```python
from build123d import *

# Parameters (mm, degrees)
SKETCH1_R                                     = 10.8
EXTRUDE1_DEPTH                                = 0.75
SKETCH2_R                                     = 10.6
EXTRUDE2_DEPTH                                = 5.5
EXTRUDE3_START                                = 5.5
SKETCH3_R                                     = 10.6
EXTRUDE3_DEPTH                                = 5.5
SKETCH4_W                                     = 16
SKETCH4_H                                     = 9
EXTRUDE4_DEPTH                                = 2
SKETCH5_W                                     = 13.3
SKETCH5_H                                     = 5.75
EXTRUDE5_DEPTH                                = 10.8
EXTRUDE6_DEPTH                                = 10.8
SKETCH7_W                                     = 10.8
SKETCH7_H                                     = 1.3
EXTRUDE7_DEPTH                                = 10.5
CHAMFER1_SIZE                                 = 0.25
SKETCH8_W                                     = 11
SKETCH8_H                                     = 12
EXTRUDE8_DEPTH                                = 13.15
EXTRUDE9_DEPTH                                = 13.15
SKETCH10_W                                    = 5.5
SKETCH10_H                                    = 3
EXTRUDE10_DEPTH                               = 13
CHAMFER2_SIZE                                 = 0.25
EXTRUDE11_DEPTH                               = 30.552834043
SKETCH12_R                                    = 10.15
EXTRUDE12_DEPTH                               = 1.25
EXTRUDE13_DEPTH                               = 13
EXTRUDE13_DEPTH_BACK                          = 5
SKETCH13_R                                    = 11.75
SKETCH13_R_2                                  = 10.15
SKETCH14_W                                    = 26
SKETCH14_H                                    = 31
SKETCH14_R                                    = 11.75
EXTRUDE14_DEPTH                               = 2
CSK_FOR_M3_COUNTERSUNK_FLAT_HEAD1_D           = 3.2
CSK_FOR_M3_COUNTERSUNK_FLAT_HEAD1_CSINK_D     = 6.3
CSK_FOR_M3_COUNTERSUNK_FLAT_HEAD1_CSINK_ANGLE = 90
FILLET1_R                                     = 3


with BuildPart() as part:
    # Sketch1 → Extrude1 (new, symmetric)
    with BuildSketch(Plane.XY):
        Circle(SKETCH1_R)
    extrude(amount=EXTRUDE1_DEPTH, both=True)

    # Sketch2 → Extrude2 (add)
    with BuildSketch(Plane.XY.offset(0.75)):
        Circle(SKETCH2_R)
    extrude(amount=EXTRUDE2_DEPTH)

    # Sketch3 → Extrude3 (add)
    with BuildSketch(Plane(origin=(0, 0, -0.75), x_dir=(-1, 0, 0), z_dir=(0, 0, -1)).offset(EXTRUDE3_START)):
        with Locations(Location((0, 0, 0), (0, 0, 180))):
            Circle(SKETCH3_R)
    extrude(amount=-EXTRUDE3_DEPTH)

    # Sketch4 → Extrude4 (add)
    with BuildSketch(Plane.XY.offset(6.25)):
        Rectangle(SKETCH4_W, SKETCH4_H)
    extrude(amount=EXTRUDE4_DEPTH)

    # Sketch5 → Extrude5 (add)
    with BuildSketch(Plane.XY.offset(8.25)):
        Rectangle(SKETCH5_W, SKETCH5_H)
    extrude(amount=EXTRUDE5_DEPTH)

    # Sketch6 → Extrude6 (cut)
    with BuildSketch(Plane.XY.offset(19.05)):
        Polygon((-5.9, 2.625), (5.9, 2.625), (6.4, 2.125), (6.4, -2.125), (5.9, -2.625), (-5.9, -2.625), (-6.4, -2.125), (-6.4, 2.125), align=None)
    extrude(amount=-EXTRUDE6_DEPTH, mode=Mode.SUBTRACT)

    # Sketch7 → Extrude7 (add)
    with BuildSketch(Plane.XY.offset(8.25)):
        with Locations((0, 0.975)):
            Rectangle(SKETCH7_W, SKETCH7_H)
    extrude(amount=EXTRUDE7_DEPTH)

    # Chamfer1
    chamfer1_edges = [part.edges().sort_by_distance(p)[0] for p in [
        (-5.4, 0.975, 18.75),
        (0, 0.325, 18.75),
        (5.4, 0.975, 18.75),
        (0, 1.625, 18.75),
    ]]
    chamfer(chamfer1_edges, length=CHAMFER1_SIZE)

    # Sketch8 → Extrude8 (add)
    with BuildSketch(Plane(origin=(0, 0, -6.25), x_dir=(-1, 0, 0), z_dir=(0, 0, -1))):
        Rectangle(SKETCH8_W, SKETCH8_H)
    extrude(amount=EXTRUDE8_DEPTH)

    # Sketch9 → Extrude9 (cut)
    with BuildSketch(Plane(origin=(0, 0, -19.4), x_dir=(-1, 0, 0), z_dir=(0, 0, -1))):
        Polygon((-2.85, 4.6), (2.85, 4.6), (3.85, 3.6), (3.85, -4.35), (-3.85, -4.35), (-3.85, 3.6), align=None)
    extrude(amount=-EXTRUDE9_DEPTH, mode=Mode.SUBTRACT)

    # Sketch10 → Extrude10 (add)
    with BuildSketch(Plane(origin=(0, 0, -6.25), x_dir=(-1, 0, 0), z_dir=(0, 0, -1))):
        Rectangle(SKETCH10_W, SKETCH10_H)
    extrude(amount=EXTRUDE10_DEPTH)

    # Chamfer2
    chamfer2_edges = [part.edges().sort_by_distance(p)[0] for p in [
        (2.75, 0, -19.25),
        (0, -1.5, -19.25),
        (-2.75, 0, -19.25),
        (0, 1.5, -19.25),
    ]]
    chamfer(chamfer2_edges, length=CHAMFER2_SIZE)

    # Sketch11 → Extrude11 (cut, through all)
    with BuildSketch(Plane(origin=(0, 0, -6.25), x_dir=(-1, 0, 0), z_dir=(0, 0, -1))):
        with BuildLine():
            Line((-2.75, 10), (-2.75, 10.444017426))
            ThreePointArc((-2.75, 10.444017426), (0, 10.8), (2.75, 10.444017426))
            Line((2.75, 10.444017426), (2.75, 10))
            ThreePointArc((2.75, 10), (0, 7.25), (-2.75, 10))
        make_face()
        with BuildLine():
            Line((-2.75, -10.444017426), (-2.75, -10))
            ThreePointArc((-2.75, -10), (0, -7.25), (2.75, -10))
            Line((2.75, -10), (2.75, -10.444017426))
            ThreePointArc((2.75, -10.444017426), (0, -10.8), (-2.75, -10.444017426))
        make_face()
    extrude(amount=-EXTRUDE11_DEPTH, mode=Mode.SUBTRACT)

    # Sketch12 → Extrude12 (add)
    with BuildSketch(Plane.XY.offset(6.25)):
        with Locations(Location((0, 0, 0), (0, 0, 105.664941507))):
            Circle(SKETCH12_R)
        Polygon((7.3, 4.8), (8.3, 4.8), (8.3, -4.8), (7.3, -4.8), (7.3, -5.25), (-7.3, -5.25), (-7.3, -4.8), (-8.3, -4.8), (-8.3, 4.8), (-7.3, 4.8), (-7.3, 5.25), (7.3, 5.25), align=None, mode=Mode.SUBTRACT)
    extrude(amount=EXTRUDE12_DEPTH)

    # Sketch13 → Extrude13 (add, two sides: drawn at the far end of the back side and taken through both)
    with BuildSketch(Plane.XY.offset(7.5).offset(-EXTRUDE13_DEPTH_BACK)):
        Circle(SKETCH13_R)
        Circle(SKETCH13_R_2, mode=Mode.SUBTRACT)
    extrude(amount=EXTRUDE13_DEPTH + EXTRUDE13_DEPTH_BACK)

    # Sketch14 → Extrude14 (add)
    with BuildSketch(Plane.XY.offset(17.65)):
        Rectangle(SKETCH14_W, SKETCH14_H)
        Circle(SKETCH14_R, mode=Mode.SUBTRACT)
    extrude(amount=-EXTRUDE14_DEPTH)

    # CSK for M3 Countersunk Flat Head1 (through all)
    with Locations(Plane.XY.offset(17.65)):
        with Locations((-9.5, 12), (9.5, -12)):
            CounterSinkHole(CSK_FOR_M3_COUNTERSUNK_FLAT_HEAD1_D / 2, CSK_FOR_M3_COUNTERSUNK_FLAT_HEAD1_CSINK_D / 2, counter_sink_angle=CSK_FOR_M3_COUNTERSUNK_FLAT_HEAD1_CSINK_ANGLE)

    # Fillet1
    fillet1_edges = [part.edges().sort_by_distance(p)[0] for p in [
        (-13, -15.5, 16.65),
        (-13, 15.5, 16.65),
        (13, 15.5, 16.65),
        (13, -15.5, 16.65),
    ]]
    fillet(fillet1_edges, radius=FILLET1_R)


solid = part.part
```
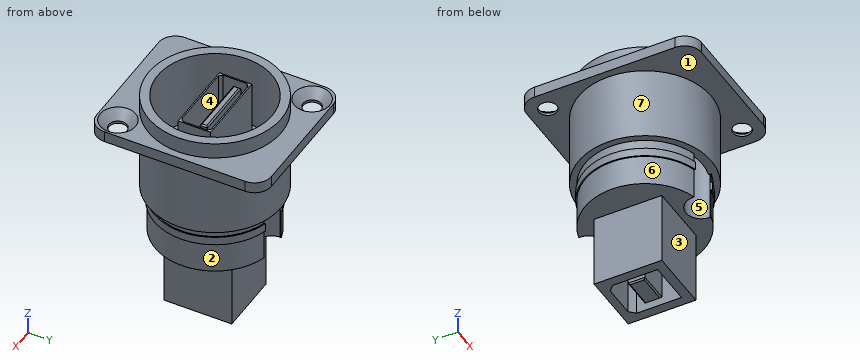
The model under review builds one solid part; all positions refer to its coordinate system, in mm. Face numbers are marked on the shaded views. A direction names the side the tool comes from. Round coordinates to 2 decimals unless told otherwise and drop trailing zeros. Order: outer loops, then holes, each group sorted by start corner. A loop starts at its lowest first (then second) coordinate and runs counter-clockwise, first axis right, second up.
(1) Take a section at A-A, the plane z = 9.5. State the section outline as (x, y) points (3 decimals).
Working result:
outline: circle Ø23.5 at (0, 0); (-6.65, -2.875) - (6.65, -2.875) - (6.65, 2.875) - (-6.65, 2.875) - close; (-5.4, 0.325) - (5.4, 0.325) - (5.4, 1.625) - (-5.4, 1.625) - close; hole circle Ø20.3 at (0, 0); hole (-6.4, -2.125) - (-5.9, -2.625) - (5.9, -2.625) - (6.4, -2.125) - (6.4, 2.125) - (5.9, 2.625) - (-5.9, 2.625) - (-6.4, 2.125) - close
(2) Take a section at B-B, the plane z = -10.5. State the section outline as (x, y) points.
Working result:
outline: (-5.5, -6) - (5.5, -6) - (5.5, 6) - (-5.5, 6) - close; (-2.75, -1.5) - (2.75, -1.5) - (2.75, 1.5) - (-2.75, 1.5) - close; hole (-3.85, -4.35) - (3.85, -4.35) - (3.85, 3.6) - (2.85, 4.6) - (-2.85, 4.6) - (-3.85, 3.6) - close
(3) For P1, Ø1.5, axis at x = 0, z = -12, coming from the -Y side; P2, Ø1.5, axis at x = 3, y = 7, coming from the +Z side; P3, Ø3, axis at x = 0, y = -9, coming from the -Z side, all flat-tipped, find the tip position at first contact; note any pin that passes through.
Working result:
P1: stops at y = -6
P2: stops at z = 7.5
P3: stops at z = 2.5
(4) Take a section at D-D, the plane y = -6.5. State the section outline as (x, z) points.
Working result:
outline: (-13, 15.65) - (-9.79, 15.65) - (-9.79, 2.5) - (-8.37, 2.5) - (-8.37, 0.75) - (-8.62, 0.75) - (-8.62, -0.75) - (-8.37, -0.75) - (-8.37, -6.25) - (8.37, -6.25) - (8.37, -0.75) - (8.62, -0.75) - (8.62, 0.75) - (8.37, 0.75) - (8.37, 2.5) - (9.79, 2.5) - (9.79, 15.65) - (13, 15.65) - (13, 17.65) - (9.79, 17.65) - (9.79, 20.5) - (7.8, 20.5) - (7.8, 7.5) - (-7.8, 7.5) - (-7.8, 20.5) - (-9.79, 20.5) - (-9.79, 17.65) - (-13, 17.65) - close
(5) Tool access review of the marked faces 1, 2, 3 and 4: name each direction out of +Z, -Z, +X, -X, +Y, -Y from which nothing blocks a thin tool from reaching the whole face with its end or side.
Working result:
face 1: -Z
face 2: -Z, +X
face 3: -Z, +X, -X, -Y
face 4: +Z
(6) Wall thickness on L1, parallel to Y at x = -0.5, z = 6.5; L2, parallel to Y at x = 1.75, z = 17.5 (3 decimals); L3, parallel to Y at x = 5, z = 7: over which ranges is each line inside the solid? List them lowest first.
Working result:
L1: y = -11.74 to -5.25, -4.5 to 4.5, 5.25 to 11.74
L2: y = -15.5 to -9.998, -2.875 to -2.625, 0.325 to 1.625, 2.625 to 2.875, 9.998 to 15.5
L3: y = -10.63 to -5.25, -4.5 to 4.5, 5.25 to 10.63
(7) Mouldability with a two-part tool opening along X and no side actions: class the marked faces 5, 6 and 7 as released by +X, released by -X, zero draft, split by the parting line, or undercut.
Working result:
face 5: undercut
face 6: released by -X
face 7: split by the parting line
